Autodesk Inventor part; units mm, degrees
ref_plane "YZ Plane" through (0, 0, 0) normal (1, 0, 0) x (0, 1, 0)
ref_plane "XZ Plane" through (0, 0, 0) normal (0, 1, 0) x (-1, 0, 0)
ref_plane "XY Plane" through (0, 0, 0) normal (0, 0, 1) x (1, 0, 0)
sketch "Sketch1" plane through (0, 0, 0) normal (0, 1, 0) x (-1, 0, 0)
  line L0 (-5, 5) -> (5, 5)
  line L1 (5, 5) -> (5, -5)
  line L2 (5, -5) -> (-5, -5)
  line L3 (-5, -5) -> (-5, 5)
  line L4 (-5, 5) -> (5, -5) construction
  line L5 (5, 5) -> (-5, -5) construction
  line L6 (-9, 9) -> (9, 9)
  line L7 (9, 9) -> (9, -9)
  line L8 (9, -9) -> (-9, -9)
  line L9 (-9, -9) -> (-9, 9)
  line L10 (-9, 9) -> (9, -9) construction
  line L11 (9, 9) -> (-9, -9) construction
  circle A0 centre (5, 5) radius 2
  circle A1 centre (-5, 5) radius 2
  circle A2 centre (5, -5) radius 2
  circle A3 centre (-5, -5) radius 2
  point P0 (0, 0)
  dimension "d0" = 10
  dimension "d1" = 10
  dimension "d2" = 18
  dimension "d3" = 18
  dimension "d4" = 4
  dimension "d5" = 4
  dimension "d6" = 4
  dimension "d7" = 4
extrude "Extrusion1" add sketch "Sketch1" along normal blind 3 contours L0 A0 L1 A2 L2 A3 L3 A1 | L6 L7 L8 L9
sketch "Sketch2" plane through (0, 3, 0) normal (0, 1, 0) x (1, 0, 0)
  line L0 (9, 9) -> (-9, 9)
  line L1 (1.5, -9) -> (-1.5, -9)
  line L2 (-1.5, -9) -> (-1.5, 9)
  line L3 (-1.5, 9) -> (1.5, 9)
  line L4 (1.5, 9) -> (1.5, -9)
  line L5 (1.5, -9) -> (-1.5, 9) construction
  line L6 (-1.5, -9) -> (1.5, 9) construction
  circle A0 centre (-5, -5) radius 2
  circle A1 centre (-5, -5) radius 4
  circle A2 centre (-5, 5) radius 2
  circle A3 centre (-5, 5) radius 4
  circle A4 centre (5, -5) radius 2
  circle A5 centre (5, -5) radius 4
  circle A6 centre (5, 5) radius 2
  circle A7 centre (5, 5) radius 4
  point P0 (0, 0)
  point P1 (1.5, -6.9365)
  point P2 (1.5, -3.0635)
  point P3 (1.5, 3.0635)
  point P4 (1.5, 6.9365)
  point P5 (-1.5, 6.9365)
  point P6 (-1.5, 3.0635)
  point P7 (-1.5, -3.0635)
  point P8 (-1.5, -6.9365)
  dimension "d10" = 3
  dimension "d11" = 8
  dimension "d12" = 8
  dimension "d13" = 8
  dimension "d14" = 8
extrude "Extrusion2" add sketch "Sketch2" along normal blind 7.6 contours L4 A7 A5 L1 L2 A1 A3 L0
sketch "Sketch3" plane through (1.5, 3, 9) normal (1, 0, 0) x (0, 0, -1)
  line L0 (0, -3) -> (0, 0)
  line L1 (0, -3) -> (0, 3.6)
  line L2 (0, 3.6) -> (18, 3.6)
  line L3 (18, 0) -> (18, 7.6)
  line L4 (18, 3.6) -> (15.5, 3.6)
  circle A0 centre (15.5, 3.6) radius 2
  circle A1 centre (15.5, 3.6) radius 4
  line L5 (19.5, -0.4) -> (11.5, -0.4)
  line L6 (11.5, -0.4) -> (11.5, 7.6)
  line L7 (11.5, 7.6) -> (19.5, 7.6)
  line L8 (19.5, 7.6) -> (19.5, -0.4)
  line L9 (19.5, -0.4) -> (11.5, 7.6) construction
  line L10 (11.5, -0.4) -> (19.5, 7.6) construction
  point P0 (9, -3)
  dimension "d17" = 6.6
  dimension "d18" = 2.5
  dimension "d19" = 4
  dimension "d20" = 8
extrude "Extrusion3" add sketch "Sketch3" against normal up to surface (3 mm away)
extrude "Extrusion4" cut sketch "Sketch3" against normal blind 10 contours L2 A0 | L2 A0
extrude "Extrusion5" cut sketch "Sketch3" along normal blind 10 contours L2 A0 | L2 A0 | A0 L2 A1 L3 | L2 L3 A1 A0 | L3 A1
extrude "Extrusion6" cut sketch "Sketch3" against normal blind 20 contours L2 A0 | L2 A0 | A0 L2 A1 L3 | L2 L3 A1 A0 | L3 A1
extrude "Extrusion7" add sketch "Sketch3" against normal up to surface (3 mm away) contours A0 L2 A1 L3 | L2 L3 A1 A0 | L3 A1
chamfer "Chamfer1" distance 13 distance2 6 1 edges at (0, 10.6, 9) measured on face at (-0.5, 10.6, -5.9788)
fillet "Fillet1" radius 2 3 edges at (0, 10.6, -10.5) (0, 2.6, -10.5) (0, 2.6, -9)
properties part number "link2"
Source: CAD feature listing. Evaluate the final solid. Frame: model axes, mm. A direction names the side the tool comes from. Round coordinates to 2 decimals unless told otherwise and drop trailing zeros. Loops run counter-clockwise (first coordinate to the right, second up) from the corner with the lowest first, then second, coordinate; pieces in that order, holes last. Notation, with made-up numbers: M 63.5,87.5 L 81.5,87.5 A17 cw 81.5,118.5 Z; hole C 33.5,49.5 d4. An arc over 180 degrees is marked long. Use a Markdown table: item, result. Add a question column.
1. Section query C-C on x = 6.5. Return the cut outline in (y, z).
2. Reachability of faces 4 (the cylindrical face through (-1, 5, 5)), 5 (the cylindrical face through (1, 5, 5)), 6 (the cylindrical face through (-3.4, 1.5, 6.2)) from +Z, -Z, +X, -X, +Y, -Y: full face, straight path, thin tool, end or side. Return the list, or none.
3. Section query D-D on z = 2.5. Return the cut outline in (x, y), then the cut area to 3 significant figures.
4. Mould query, pull axis Y, two halves, no side actions, for faces 1 (the cylindrical face through (0, 5.4, -4.9)), 2 (the flat face through (1.5, 4, 8)), 3 (the flat face through (0, 0, 0)). Classes: pulls with the +Y half, pulls with the -Y half, needs draft (parallel to the pull), parting line crosses it, or undercut.
5. Line query: line 1 (Z direction, x = 5, y = 0.7); line 2 (Y direction, x = -0.4, z = -6.5). Output: solid intervals per line, ascending.
6. Section query B-B on z = 6.5. Return the cut outline in (x, y), then the cut area to 3 significant figures.
7. Section query A-A on x = 0.5. Return the cut outline in (y, z), then the cut area to 3 significant figures.
8. Contact query for flat-ended pins moving along their axis: P1, Ø0.6, axis at y = 4.5, z = 7.5, coming from the -X side; P2, Ø0.6, axis at y = 4, z = 7.5, coming from the +X side; P3, Ø0.6, axis at x = -4, z = -8.5, coming from the +Y side. Output: stop coordinate, or through.
Reported:
| question | item | result |
|---|---|---|
| 1 | outline | M 0,-9 L 3,-9 L 3,-8.24 A4 cw 2.6,-6.32 L 0,-6.32 Z; M 0,-3.68 L 3,-3.68 L 3,3.68 L 0,3.68 Z; M 0,6.32 L 3,6.32 L 3,9 L 0,9 Z |
| 2 | face 4 | -X, +Y |
| 2 | face 5 | +X, +Y |
| 2 | face 6 | +Y, -Y |
| 3 | outline | M -9,0 L 9,0 L 9,3 L 1.5,3 L 1.5,7.6 L -1.5,7.6 L -1.5,3 L -9,3 Z |
| 3 | area | 67.8 mm² |
| 4 | face 1 | undercut |
| 4 | face 2 | needs draft |
| 4 | face 3 | pulls with the -Y half |
| 5 | line 1 | z = -9 to -7, -3 to 3, 7 to 9 |
| 5 | line 2 | y = 0 to 4.6, 8.6 to 10.6 |
| 6 | outline | M -9,0 L -6.32,0 L -6.32,3 L -9,3 Z; M -3.68,0 L 3.68,0 L 3.68,3 L 1.29,3 L 1.29,5.75 L -1.29,5.75 L -1.29,3 L -3.68,3 Z; M 6.32,0 L 9,0 L 9,3 L 6.32,3 Z |
| 6 | area | 45.2 mm² |
| 7 | outline | M 0,-9 L 0.66,-9 A2 cw 2.22,-9.75 A2 ccw 3.79,-10.5 L 8.6,-10.5 A2 ccw 10.6,-8.5 L 10.6,-4 L 4.6,9 L 0,9 Z; hole C 6.6,-6.5 d4 |
| 7 | area | 151 mm² |
| 8 | P1 | stops at x = -1.5 |
| 8 | P2 | stops at x = 1.5 |
| 8 | P3 | stops at y = 3 |
